Autodesk Inventor part; units mm, degrees
ref_plane "YZ Plane" through (0, 0, 0) normal (1, 0, 0) x (0, 1, 0)
ref_plane "XZ Plane" through (0, 0, 0) normal (0, 1, 0) x (-1, 0, 0)
ref_plane "XY Plane" through (0, 0, 0) normal (0, 0, 1) x (1, 0, 0)
sketch "Sketch1" plane through (0, 0, 0) normal (0, 0, 1) x (1, 0, 0)
  line L0 (0, 0) -> (60.452, 0)
  line L1 (60.452, 0) -> (60.452, 30.988)
  line L2 (60.452, 30.988) -> (0, 30.988)
  line L3 (0, 30.988) -> (0, 0)
  dimension "d0" = 60.452
  dimension "d1" = 30.988
extrude "Extrusion1" add sketch "Sketch1" along normal blind 23.368
sketch "Sketch2" plane through (60.452, 0, 0) normal (1, 0, 0) x (0, 0, -1)
  line L0 (-4.699, 30.988) -> (-18.669, 30.988)
  line L1 (-18.669, 30.988) -> (-18.669, 34.163)
  line L2 (-18.669, 34.163) -> (-4.699, 34.163)
  line L3 (-4.699, 34.163) -> (-4.699, 30.988)
  line L4 (0, 30.988) -> (-23.368, 30.988)
  point P0 (0, 0)
  point P1 (-11.684, 34.163)
  point P2 (-11.684, 30.988)
  point P3 (-11.684, 30.988)
  dimension "d4" = 13.97
  dimension "d5" = 3.175
extrude "Extrusion2" add sketch "Sketch2" along normal blind 8.89 and the other way blind 6.35
fillet "Fillet1" radius 3.175 3 edges at (54.102, 30.988, 11.684) (57.277, 30.988, 18.669) (57.277, 30.988, 4.699)
properties part number "ASDSBattery" material "ABS Plastic"
Verification items for the finished model (mm, model axes). A direction names the side the tool comes from. Give positions to 0.01 mm unless a question says otherwise; leave off trailing zeros. Loops run counter-clockwise (first coordinate to the right, second up) from the corner with the lowest first, then second, coordinate; pieces in that order, holes last.
1. Thickness scan on line 1 (Y direction, x = 31, z = 20.75); line 2 (X direction, y = 22, z = 18); line 3 (Y direction, x = 61, z = 5.5). Record the ranges inside material, lowest first.
2. Section check B-B, the plane x = 42. Enter the section's corners in (y, z).
3. Go/stop test with flat-tipped pins: pin 1 Ø10 at (x, z) = (63, 11.5) entering from -Y; pin 2 Ø1 at (x, z) = (44.5, 12.5) entering from +Y; pin 3 Ø2.5 at (x, y) = (62, 32.5) entering from +Z; pin 4 Ø3.5 at (x, y) = (61, 33) entering from -Z. Record where each tip stops, or that it passes through.
4. Section check D-D, the plane y = 32.5. Enter the section's corners in (x, z).
5. Set-up check for faces 1 (the cylindrical face through (53.147, 31.893, 11.826)), 2 (the flat face through (65, 33, 4.699)), 3 (the flat face through (65, 30.988, 12)): record each of +Z, -Z, +X, -X, +Y, -Y from which the full face is reachable in a straight line by a thin tool's end or side.
6. Section check C-C, the plane y = 20.5. Enter the section's corners in (x, z).
Geometry says:
1. line 1: y = 0 to 30.99
1. line 2: x = 0 to 60.45
1. line 3: y = 30.99 to 34.16
2. outline: (0, 0) - (30.99, 0) - (30.99, 23.37) - (0, 23.37) - close
3. pin 1: stops at y = 0
3. pin 2: stops at y = 30.99
3. pin 3: stops at z = 18.67
3. pin 4: stops at z = 2.97
4. outline: (53.63, 4.23) - (60.45, 4.23) - (60.45, 4.7) - (69.34, 4.7) - (69.34, 18.67) - (60.45, 18.67) - (60.45, 19.14) - (53.63, 19.14) - close
5. face 1: +Z, -Z, -X, +Y
5. face 2: -Z, +X, +Y, -Y
5. face 3: +Z, -Z, +X, -Y
6. outline: (0, 0) - (60.45, 0) - (60.45, 23.37) - (0, 23.37) - close
